Model file for the job. Use its own axes, mm. A direction names the side the tool comes from. Coordinates: 2 decimals unless noted, no trailing zeros. Write each loop counter-clockwise with the first axis right and the second up, starting at its lowest first coordinate (ties: lowest second). Pieces come first, ordered by that corner, then holes. Notation, with made-up numbers: M -20,43.5 L -2,43.5 A26 cw -2,64.5 Z; hole C -1,79.5 d1. An arc over 180 degrees is marked long. Put each result on its own line as item: value. Start each with the question number.
Q1. Pull direction Y, two halves, no side cores. Call faces 1 (the flat face through (-263.75, 0, 1)), 2 (the flat face through (4, -10, 7)), 3 (the flat face through (4, -12.5, 8)): pulls with the +Y half, pulls with the -Y half, needs draft (parallel to the pull), parting line crosses it, or undercut.
Q2. Cut at B-B (x = -5). Write the cut outline in (y, z).
Q3. Drill centre lines: line 1 along Z through (x, y) = (222.5, -6.5); line 2 along Y through (x, z) = (80, 7.25); line 3 along Z through (x, y) = (-128, -2.5). Where is each one in solid material? Low to high.
Q4. Drop a flat-ended pin along its axis: pin 1 (1.5 mm diameter, centred on y = 3.5, z = 5, fed in from +X). Give the stop position or say it passes through.
Q5. Which spindle directions (+Z, -Z, +X, -X, +Y, -Y) get a long thin tool onto all of the face, cutting with end or side? Do faces 4 (the flat face through (4, 12.5, 7)), 5 (the flat face through (4, 0, 2.5)). Say none if no direction does.
Q6. Cut at A-A (z = 9). Write the cut outline in (x, y), then the cut area to 3 significant figures.
```python
from build123d import *

# Parameters (mm, degrees)
F1_DEPTH = 263.75


with BuildPart() as f1:
    # F0 (on Right) → F1 (new body, symmetric)
    with BuildSketch(Plane.YZ):
        Polygon((-10, 15), (-12.5, 15), (-12.5, 12.5), (-12.5, 0), (12.5, 0), (12.5, 12.5), (12.5, 15), (10, 15), (5.2, 15), (5.2, 12.5), (10, 12.5), (10, 2.5), (-10, 2.5), (-10, 12.5), (-5.2, 12.5), (-5.2, 15), align=None)
    extrude(amount=F1_DEPTH, both=True)


solid = f1.part
```
Computed values:
1. face 1: needs draft
1. face 2: undercut
1. face 3: pulls with the -Y half
2. outline: M -12.5,0 L 12.5,0 L 12.5,15 L 5.2,15 L 5.2,12.5 L 10,12.5 L 10,2.5 L -10,2.5 L -10,12.5 L -5.2,12.5 L -5.2,15 L -12.5,15 Z
3. line 1: 0 to 2.5, 12.5 to 15
3. line 2: -12.5 to -10, 10 to 12.5
3. line 3: 0 to 2.5
4. pin 1: through
5. face 4: +Z, -Z, +X, -X, +Y
5. face 5: +X, -X
6. outline: M -263.75,-12.5 L 263.75,-12.5 L 263.75,-10 L -263.75,-10 Z; M -263.75,10 L 263.75,10 L 263.75,12.5 L -263.75,12.5 Z
6. area: 2,640 mm2
